Autodesk Inventor part; units mm, degrees
ref_plane "YZ Plane" through (0, 0, 0) normal (1, 0, 0) x (0, 1, 0)
ref_plane "XZ Plane" through (0, 0, 0) normal (0, 1, 0) x (-1, 0, 0)
ref_plane "XY Plane" through (0, 0, 0) normal (0, 0, 1) x (1, 0, 0)
sketch "スケッチ1" plane through (0, 0, 0) normal (0, 0, 1) x (1, 0, 0)
  circle A0 centre (0, 0) radius 5
  circle A1 centre (0, 50) radius 5
  arc A2 (11.6485, 45.4655) -> (-11.6485, 45.4655) centre (0, 50) ccw
  arc A3 (-11.6485, 4.5345) -> (11.6485, 4.5345) centre (0, 0) ccw
  circle A4 centre (0, 30) radius 1.6
  circle A5 centre (0, 30) radius 8 construction
  arc A6 (-11.6485, 4.5345) -> (-11.6485, 45.4655) centre (-64.2223, 25) ccw
  arc A7 (11.6485, 45.4655) -> (11.6485, 4.5345) centre (64.2223, 25) ccw
  dimension "d0" = 10
  dimension "d1" = 10
  dimension "d2" = 50
  dimension "d3" = 12.5
  dimension "d4" = 12.5
  dimension "d11" = 3.2
  dimension "d12" = 20
  dimension "d13" = 16
extrude "押し出し1" add sketch "スケッチ1" along normal blind 4
sketch "スケッチ2" plane through (0, 0, 4) normal (0, 0, 1) x (1, 0, 0)
  circle A0 centre (0, 0) radius 11.05
  circle A1 centre (0, 50) radius 5
  circle A2 centre (0, 50) radius 11.05
  dimension "d7" = 22.1
  dimension "d8" = 22.1
extrude "押し出し2" cut sketch "スケッチ2" against normal blind 3
properties part number "ハンド_リンク1" material "アルミニウム 6061"
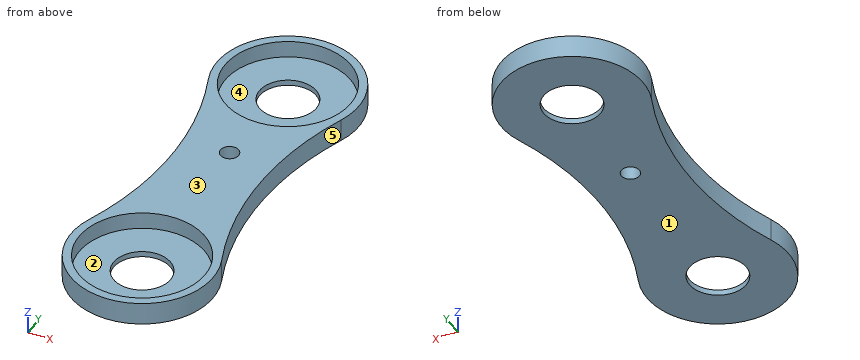
Input: part model. Units: mm. Frame: model coordinates. Face numbers are marked on the shaded views. A direction names the side the tool comes from. Coordinates: 2 decimals unless noted, no trailing zeros. Loops run counter-clockwise (first coordinate to the right, second up) from the corner with the lowest first, then second, coordinate; pieces in that order, holes last. Notation, with made-up numbers: (48.25, 0) -> (53.25, 0) arc R6 cw to (53.25, 4) -> close; hole circle Ø9 at (-26, -17.75). An arc over 180 degrees is marked (long way). Write each question's results on one line, items separated by ' | '. Start each with the question number.
Q1. Section A-A, the plane y = 0. Return the cut outline in (x, z).
Q2. Pull-direction query (X, two-part tool) for the marked faces 3, 4 and 5; classes: released by +X, released by -X, zero draft, split by the parting line, or undercut.
Q3. Pin query (flat end, axial travel): pin 1 (9 mm diameter, centred on x = 0, y = 50, fed in from +Z); pin 2 (3 mm diameter, centred on x = 0, y = -4, fed in from +Z); pin 3 (1 mm diameter, centred on y = 39, z = 1, fed in from -X). Return the tip coordinate at first contact, or that it passes through.
Q4. Ray query, line 1 (Y direction, x = 0.5, z = 2.65); line 2 (X direction, y = 0, z = 0.25); line 3 (Y direction, x = -1.75, z = 2.8). Return the intervals inside material, ascending. Write a range as from..to.
Q5. Section B-B, the plane z = 2.15. Return the cut outline in (x, y).
Q6. Section D-D, the plane x = 4. Return the cut outline in (y, z), plus the area to 3 significant figures.
Q7. Section C-C, the plane x = 0. Return the cut outline in (y, z).
Q8. Reachability of the marked faces 1 and 2 from +Z, -Z, +X, -X, +Y, -Y: full face, straight path, thin tool, end or side. Return the list, or none.
Found:
1) outline: (-12.5, 0) -> (-5, 0) -> (-5, 1) -> (-11.05, 1) -> (-11.05, 4) -> (-12.5, 4) -> close; (5, 0) -> (12.5, 0) -> (12.5, 4) -> (11.05, 4) -> (11.05, 1) -> (5, 1) -> close
2) face 3: zero draft | face 4: undercut | face 5: released by +X
3) pin 1: through | pin 2: z = 1 | pin 3: x = -9.7
4) line 1: -12.49..-11.04, 11.04..28.48, 31.52..38.96, 61.04..62.49 | line 2: -12.5..-5, 5..12.5 | line 3: -12.38..-10.91, 10.91..39.09, 60.91..62.38
5) outline: (-11.65, 4.53) arc R12.5 ccw (long way) to (11.65, 4.53) arc R56.42 cw to (11.65, 45.47) arc R12.5 ccw (long way) to (-11.65, 45.47) arc R56.42 cw to start; hole circle Ø22.1 at (0, 0); hole circle Ø22.1 at (0, 50); hole circle Ø3.2 at (0, 30)
6) outline: (-11.84, 0) -> (-3, 0) -> (-3, 1) -> (-10.3, 1) -> (-10.3, 4) -> (-11.84, 4) -> close; (3, 0) -> (47, 0) -> (47, 1) -> (39.7, 1) -> (39.7, 4) -> (10.3, 4) -> (10.3, 1) -> (3, 1) -> close; (53, 0) -> (61.84, 0) -> (61.84, 4) -> (60.3, 4) -> (60.3, 1) -> (53, 1) -> close | area: 159 mm2
7) outline: (-12.5, 0) -> (-5, 0) -> (-5, 1) -> (-11.05, 1) -> (-11.05, 4) -> (-12.5, 4) -> close; (5, 0) -> (28.4, 0) -> (28.4, 4) -> (11.05, 4) -> (11.05, 1) -> (5, 1) -> close; (31.6, 0) -> (45, 0) -> (45, 1) -> (38.95, 1) -> (38.95, 4) -> (31.6, 4) -> close; (55, 0) -> (62.5, 0) -> (62.5, 4) -> (61.05, 4) -> (61.05, 1) -> (55, 1) -> close
8) face 1: -Z, +X, -X, +Y, -Y | face 2: +Z
